```python
from build123d import *

# Parameters (mm, degrees)
F1_DEPTH       = 10
F3_D           = 4.5
F3_CSINK_D     = 8.5
F3_CSINK_ANGLE = 90
F4_SIZE        = 1


with BuildPart() as f1:
    # F0 (on Top) → F1 (new body)
    with BuildSketch(Plane.XY):
        Polygon((60, 0), (0, 0), (0, -5), (10, -5), (10, -30), (50, -30), (50, -10), (45, -10), (45, -25), (15, -25), (15, -5), (60, -5), align=None)
    extrude(amount=F1_DEPTH)

    # F3 (through all)
    with Locations(Plane.XZ.offset(5)):
        with Locations((5, 5), (55, 5)):
            CounterSinkHole(F3_D / 2, F3_CSINK_D / 2, counter_sink_angle=F3_CSINK_ANGLE)

    # F4
    f4_edges = [f1.edges().sort_by_distance(p)[0] for p in [
        (50, -10, 5),
        (45, -10, 5),
        (15, -5, 5),
        (15, -25, 5),
        (45, -25, 5),
        (50, -30, 5),
        (10, -30, 5),
    ]]
    chamfer(f4_edges, length=F4_SIZE)


solid = f1.part
```
Part model, mm, in its own coordinate system. A direction names the side the tool comes from. Coordinates: 2 decimals unless noted, no trailing zeros. Write each loop counter-clockwise with the first axis right and the second up, starting at its lowest first coordinate (ties: lowest second). Pieces come first, ordered by that corner, then holes.
Item 1: Slice it at D-D (x = 23). Write the cut outline in (y, z), and give its area (3 significant figures).
Item 2: Slice it at A-A (z = 5). Count the separate pieces of the cut face and the enclosed holes in it, and give its area (4 significant figures).
Item 3: Slice it at B-B (x = 55). Write the cut outline in (y, z).
Item 4: Mould opens along Y. For faces 1 (the face through (0, -2, 5)), 2 (the face through (15, -15, 5)), 3 (the face through (0.5, -5, 4.9)) say: released by +Y, released by -Y, zero draft, split by the parting line, or undercut.
Item 5: Probe line 1 (X direction, y = -1.1, z = 5); line 2 (Y direction, x = 24.5, z = 0.75); line 3 (X direction, y = -3.25, z = 7). List the from-to ranges inside material, lowest first.
Item 6: Which spindle directions (+Z, -Z, +X, -X, +Y, -Y) get a long thin tool onto all of the face, cutting with end or side? Do faces 4 (the face through (50, -20, 5)), 5 (the face through (30, -30, 5)), 6 (the face through (30, -25, 5)), 7 (the face through (10, -17, 5)), 8 (the face through (33, -5, 5)). Say none if no direction does.
Item 7: Pin check, flat tips, straight feed: pin 1 (2 mm diameter, centred on y = -16, z = 5, fed in from -X); pin 2 (3 mm diameter, centred on x = 7.5, z = 3, fed in from -Y). Stop position of each tip, or through.
Item 8: Slice it at C-C (y = -13.5). Write the cut outline in (x, z), and give its area (3 significant figures).
Results found:
1. outline: (-30, 0) - (-25, 0) - (-25, 10) - (-30, 10) - close; (-5, 0) - (0, 0) - (0, 10) - (-5, 10) - close
1. area: 100 mm2
2. separate pieces: 3
2. enclosed holes: 0
2. area: 621.5 mm2
3. outline: (-5, 0) - (0, 0) - (0, 2.75) - (-3, 2.75) - (-5, 0.75) - close; (-5, 9.25) - (-3, 7.25) - (0, 7.25) - (0, 10) - (-5, 10) - close
4. face 1: zero draft
4. face 2: undercut
4. face 3: released by -Y
5. line 1: x = 0 to 2.75, 7.25 to 52.75, 57.25 to 60
5. line 2: y = -30 to -25, -5 to 0
5. line 3: x = 0 to 3.5, 6.5 to 53.5, 56.5 to 60
6. face 4: +Z, -Z, +X, -Y
6. face 5: +Z, -Z, +X, -X, -Y
6. face 6: +Z, -Z
6. face 7: +Z, -Z, -X, -Y
6. face 8: +Z, -Z, +X
7. pin 1: stops at x = 10
7. pin 2: stops at y = -5
8. outline: (10, 0) - (15, 0) - (15, 10) - (10, 10) - close; (45, 0) - (50, 0) - (50, 10) - (45, 10) - close
8. area: 100 mm2
